from build123d import *

# Parameters (mm, degrees)
CHAMFER_1_SIZE = 0.5


with BuildPart() as part:
    # 草图1 → 旋转1 (revolve)
    with BuildSketch(Plane.XY):
        Polygon((-13.5, 4.975), (13.5, 4.975), (13.5, 6.025), (10, 6.025), (10, 7), (-10, 7), (-10, 6.025), (-13.5, 6.025), align=None)
    revolve(axis=Axis((13.5, 0, 0), (-1, 0, 0)))

    # 倒角1
    chamfer_1_edges = [part.edges().sort_by_distance(p)[0] for p in [
        (-13.5, -6.025, 0),
        (13.5, -6.025, 0),
        (10, -7, 0),
        (-10, -7, 0),
    ]]
    chamfer(chamfer_1_edges, length=CHAMFER_1_SIZE)


solid = part.part
Verification items for the finished model (mm, model axes). A direction names the side the tool comes from. Coordinates: 2 decimals unless noted, no trailing zeros. Loops run counter-clockwise (first coordinate to the right, second up) from the corner with the lowest first, then second, coordinate; pieces in that order, holes last. Notation, with made-up numbers: (66.25, 34) -> (73.25, 34) arc R24 cw to (73.25, 57) -> close; hole circle Ø10 at (-1.75, 69). An arc over 180 degrees is marked (long way). Answer as a JSON object with one key per item and string values. Group by question number.
Item 1: Mould release check, pull along Z, two halves, no side actions. Record for faces 1 (the flat face through (-10, 2, 6)), 2 (the cylindrical face through (0.189, -3.948, 3.027)), 3 (the cylindrical face through (-0.133, 6.466, 2.681)): +Z half, -Z half, draft (parallel to the pull), parting line (faces both ways), or undercut.
Item 2: Sectioned sample at A-A on y = 0. Record the boundary of the cut face in (x, z) (3 decimals).
Item 3: Depth check by flat-ended pin: pin 1 (3 mm diameter, centred on x = 7.5, z = 5, fed in from -Y); pin 2 (3 mm diameter, centred on x = 10, y = 5, fed in from -Z). Enter the tip coordinate at first touch or a pass-through.
Item 4: Tool access check on faces 4 (the cylindrical face through (11.48, -4.44, -4.07)), 5 (the cylindrical face through (-11.52, -4.44, -4.07)). Record the directions out of +Z, -Z, +X, -X, +Y, -Y that give a thin tool (end or side, any length) a straight path to the whole face; none if there is none.
Item 5: Sectioned sample at C-C on x = 1.75. Record the boundary of the cut face in (y, z) (3 decimals), plus the area to 3 significant figures.
Item 6: Scan lines: probe 1 along Z at (x, y) = (6, 0) (3 decimals); probe 2 along Z at (x, y) = (-1.25, 1.5). Record each from-to range of solid material in increasing order.
Evaluation:
{
 "1": {"face 1": "draft", "face 2": "undercut", "face 3": "parting line"},
 "2": {"outline": "(-13.5, -5.525) -> (-13, -6.025) -> (-10, -6.025) -> (-10, -6.5) -> (-9.5, -7) -> (9.5, -7) -> (10, -6.5) -> (10, -6.025) -> (13, -6.025) -> (13.5, -5.525) -> (13.5, -4.975) -> (-13.5, -4.975) -> close; (-13.5, 4.975) -> (13.5, 4.975) -> (13.5, 5.525) -> (13, 6.025) -> (10, 6.025) -> (10, 6.5) -> (9.5, 7) -> (-9.5, 7) -> (-10, 6.5) -> (-10, 6.025) -> (-13, 6.025) -> (-13.5, 5.525) -> close"},
 "3": {"pin 1": "stops at y = -6.06", "pin 2": "stops at z = -6.01"},
 "4": {"face 4": "+X", "face 5": "-X"},
 "5": {"outline": "circle Ø14 at (0, 0); hole circle Ø9.95 at (0, 0)", "area": "76.2 mm²"},
 "6": {"probe 1": "z = -7 to -4.975, 4.975 to 7", "probe 2": "z = -6.84 to -4.74, 4.74 to 6.84"}
}
